Verification items for this drawing (mm, ordinates from the low corner). Coordinates: 2 decimals unless noted, no trailing zeros. Write each loop counter-clockwise with the first axis right and the second up, starting at its lowest first coordinate (ties: lowest second). Pieces come first, ordered by that corner, then holes. Notation, with made-up numbers: (57, -22) -> (110, -22) arc R18 cw to (110, -18) -> close; hole circle Ø10 at (-24.5, -11). An arc over 180 degrees is marked (long way). One line per item, written item: value. Start each with the question number.
1) Sectioned sample at A-A on z = 3. Enter the section's corners in (x, y), plus the area to 3 significant figures.
2) Sectioned sample at B-B on y = 2.45. Enter the section's corners in (x, z).
3) Gauge pin test, flat ends, axial feed: P1, Ø1.3, axis at x = 3.5, y = 2.5, coming from the -Z side; P2, Ø1.3, axis at y = 2.5, z = 28, coming from the +X side; P3, Ø0.8, axis at y = 2.5, z = 28.5, coming from the -X side. Record the tip position at first contact, or that the pin passes through.
4) Scan lines: line 1 along Y through (x, z) = (2.5, 5.5); line 2 along Z through (x, y) = (3.5, 2.5); line 3 along X through (y, z) = (0.1, 16) (1 decimal). Record each from-to range of solid material in increasing order. Write a range as [from, to].
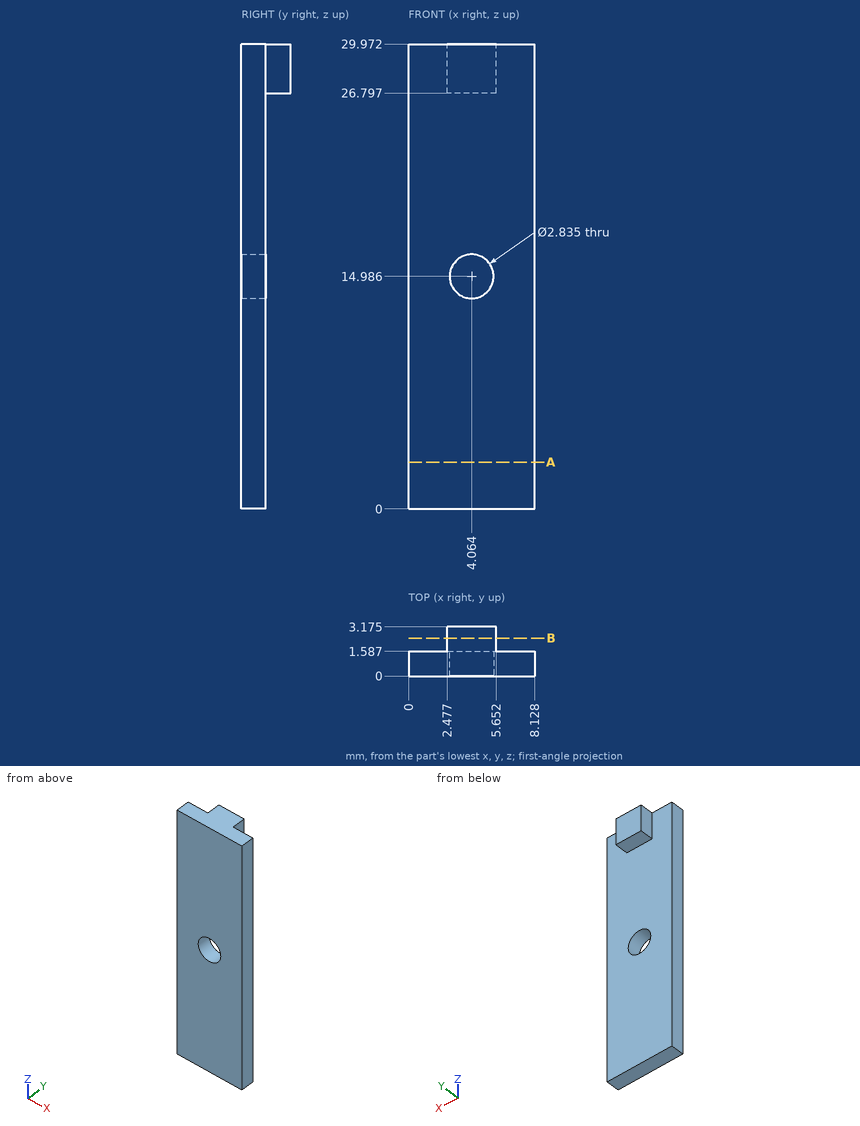
Answers:
1. outline: (0, 0) -> (8.13, 0) -> (8.13, 1.59) -> (0, 1.59) -> close
1. area: 12.9 mm2
2. outline: (2.48, 26.8) -> (5.65, 26.8) -> (5.65, 29.97) -> (2.48, 29.97) -> close
3. P1: stops at z = 26.8
3. P2: stops at x = 5.65
3. P3: stops at x = 2.48
4. line 1: y = [0, 1.59]
4. line 2: z = [26.8, 29.97]
4. line 3: x = [0, 3.1], [5.1, 8.1]
